from build123d import *

# Parameters (mm, degrees)
SKETCH1_W           = 139.7
SKETCH1_H           = 439.61
BOSS_EXTRUDE1_DEPTH = 2
SKETCH2_W           = 139.7
SKETCH2_H           = 2
BOSS_EXTRUDE2_DEPTH = 15.24
FILLET1_R           = 1.5
FILLET2_R           = 0.5


with BuildPart() as part:
    # Sketch1 → Boss-Extrude1 (new body)
    with BuildSketch(Plane(origin=(0, 0, 0), x_dir=(1, 0, 0), z_dir=(0, 1, 0))):
        with Locations((-225.481193932, 42.830702244)):
            Rectangle(SKETCH1_W, SKETCH1_H)
    extrude(amount=BOSS_EXTRUDE1_DEPTH)

    # Sketch2 → Boss-Extrude2 (add)
    with BuildSketch(Plane.XZ):
        with Locations((-225.481193932, -261.635702244)):
            Rectangle(SKETCH2_W, SKETCH2_H)
        with Locations((-225.481193932, 175.974297756)):
            Rectangle(SKETCH2_W, SKETCH2_H)
    extrude(amount=BOSS_EXTRUDE2_DEPTH)

    # Fillet1
    fillet1_edges = [part.edges().sort_by_distance(p)[0] for p in [
        (-225.481193932, 2, 176.974297756),
        (-225.481193932, 2, -262.635702244),
    ]]
    fillet(fillet1_edges, radius=FILLET1_R)

    # Fillet2
    fillet2_edges = [part.edges().sort_by_distance(p)[0] for p in [
        (-225.481193932, 0, -260.635702244),
        (-225.481193932, 0, 174.974297756),
    ]]
    fillet(fillet2_edges, radius=FILLET2_R)


solid = part.part
CAD build for the part. Positions are in the model's coordinates, mm. A direction names the side the tool comes from. Round coordinates to 2 decimals unless told otherwise and drop trailing zeros. Loops run counter-clockwise (first coordinate to the right, second up) from the corner with the lowest first, then second, coordinate; pieces in that order, holes last.
(1) Cut at B-B (x = -214.5). Give the cut face in (y, z), plus the area to 3 significant figures.
(2) Drop a flat-ended pin along its axis: pin 1 (8 mm diameter, centred on y = -7.5, z = -90.5, fed in from +X). Give the stop position or say it passes through.
(3) Two-plate mould, pull along Z, no slides. Class faces 1 (the flat face through (-226, -7, 176.974)), 2 (the flat face through (-155.631, 1, -44)), 3 (the flat face through (-226, -8, -260.636)), 4 (the flat face through (-226, -7, -262.636)): +Z half, -Z half, draft (parallel to the pull), parting line (faces both ways), or undercut.
(4) Which spindle directions (+Z, -Z, +X, -X, +Y, -Y) get a long thin tool onto all of the face, cutting with end or side? Do faces 5 (the flat face through (-226, -8, 174.974)), 6 (the flat face through (-295.331, 1, -44)). Say none if no direction does.
(5) Cut at C-C (z = -141). Give the cut face in (x, y).
(6) Cut at A-A (y = -6). Give the cut face in (x, z), plus the area to 3 significant figures.
(7) Wall check: line 1 along Z through (x, y) = (-237, -8); line 2 along Z through (x, y) = (-182, 0.75); line 3 along Y through (x, z) = (-274, -124.5). Give the ranges that are in metal, low to high.
Findings below:
1. outline: (-15.24, -262.64) - (0.5, -262.64) arc R1.5 ccw to (2, -261.14) - (2, 175.47) arc R1.5 ccw to (0.5, 176.97) - (-15.24, 176.97) - (-15.24, 174.97) - (-0.5, 174.97) arc R0.5 cw to (0, 174.47) - (0, -260.14) arc R0.5 cw to (-0.5, -260.64) - (-15.24, -260.64) - close
1. area: 939 mm2
2. pin 1: passes through
3. face 1: +Z half
3. face 2: draft
3. face 3: undercut
3. face 4: -Z half
4. face 5: +X, -X, -Y
4. face 6: +Z, -Z, -X, +Y, -Y
5. outline: (-295.33, 0) - (-155.63, 0) - (-155.63, 2) - (-295.33, 2) - close
6. outline: (-295.33, -262.64) - (-155.63, -262.64) - (-155.63, -260.64) - (-295.33, -260.64) - close; (-295.33, 174.97) - (-155.63, 174.97) - (-155.63, 176.97) - (-295.33, 176.97) - close
6. area: 559 mm2
7. line 1: z = -262.64 to -260.64, 174.97 to 176.97
7. line 2: z = -262.61 to 176.95
7. line 3: y = 0 to 2
